from build123d import *

# Parameters (mm, degrees)
F0_W     = 250
F0_H     = 250
F1_DEPTH = 250
F3_DEPTH = 25
F4_R     = 1.5
F5_DEPTH = 70


with BuildPart() as f1:
    # F0 (on Top) → F1 (new body)
    with BuildSketch(Plane.XY):
        with Locations((62.549456, 79.716726)):
            Rectangle(F0_W, F0_H)
    extrude(amount=F1_DEPTH)

    # F2 (on face) → F3 (join)
    with BuildSketch(Plane.XY.offset(250)):
        Polygon((37.549456, -45.283274), (62.549456, -45.283274), (87.549456, -45.283274), (87.549456, -20.283274), (37.549456, -20.283274), align=None)
    extrude(amount=F3_DEPTH)

    # F4 (on face) → F5 (cut)
    with BuildSketch(Plane.XZ.offset(45.283274)):
        with Locations((62.549456, 244)):
            Circle(F4_R)
    extrude(amount=-F5_DEPTH, mode=Mode.SUBTRACT)


solid = f1.part
Source: CAD feature listing. Evaluate the final solid. Frame: model axes, mm. A direction names the side the tool comes from. Round coordinates to 2 decimals unless told otherwise and drop trailing zeros. Write each loop counter-clockwise with the first axis right and the second up, starting at its lowest first coordinate (ties: lowest second). Pieces come first, ordered by that corner, then holes. Notation, with made-up numbers: M -8.75,52 L 27.25,52 A24 cw 27.25,76 Z; hole C -1.5,-20 d5. An arc over 180 degrees is marked long. One line per item, written item: value. Start each with the question number.
Item 1: Set-up query: faces 1 (the flat face through (87.549, -33, 262)), 2 (the flat face through (63, -20.283, 262)), 3 (the flat face through (37.549, -33, 262)), 4 (the flat face through (61, 204.717, 123)). Return all of +Z, -Z, +X, -X, +Y, -Y with unobstructed straight access to the full face (end or side cutting, diameter ignored); none if empty.
Item 2: Section query C-C (y = 82). Return the cut outline in (x, z), plus the area to 3 significant figures.
Item 3: Section query B-B (x = -30.5). Return the cut outline in (y, z), plus the area to 3 significant figures.
Item 4: Pin query (flat end, axial travel): pin 1 (12 mm diameter, centred on x = 155.5, y = 115, fed in from +Z); pin 2 (12.5 mm diameter, centred on x = 63.5, z = 266.5, fed in from +Y); pin 3 (1.5 mm diameter, centred on x = 90.5, y = 9, fed in from -Z). Return the tip coordinate at first contact, or that it passes through.
Item 5: Section query A-A (y = -0.5). Return the cut outline in (x, z), plus the area to 3 significant figures.
Item 6: Ray query, L1, parallel to X at y = -21.5, z = 244; L2, parallel to Z at x = 70, y = 144.5. Return the intervals inside material, ascending. Write a range as from..to.
Result set:
1. face 1: +Z, +X, +Y, -Y
1. face 2: +Z, +X, -X, +Y
1. face 3: +Z, -X, +Y, -Y
1. face 4: +Z, -Z, +X, -X, +Y
2. outline: M -62.45,0 L 187.55,0 L 187.55,250 L -62.45,250 Z
2. area: 62,500 mm²
3. outline: M -45.28,0 L 204.72,0 L 204.72,250 L -45.28,250 Z
3. area: 62,500 mm²
4. pin 1: stops at z = 250
4. pin 2: stops at y = -20.28
4. pin 3: stops at z = 0
5. outline: M -62.45,0 L 187.55,0 L 187.55,250 L -62.45,250 Z; hole C 62.55,244 d3
5. area: 62,500 mm²
6. L1: x = -62.45..61.05, 64.05..187.55
6. L2: z = 0..250
